Can you work these out from the model? Positions are in its coordinate system, mm. A direction names the side the tool comes from. Coordinates: 2 decimals unless noted, no trailing zeros. Loops run counter-clockwise (first coordinate to the right, second up) from the corner with the lowest first, then second, coordinate; pieces in that order, holes last. Notation, with made-up numbers: (49.5, -4) -> (70.5, -4) arc R18 ccw to (70.5, 29) -> close; hole circle Ø5 at (30.5, 79.25). An arc over 180 degrees is marked (long way). Use one line per item in the form item = value. Start each with the question number.
(1) I'm going to push flat-ended pins straight in: pin 1 (1.2 mm diameter, centred on y = 7, z = 9, fed in from -X); pin 2 (3 mm diameter, centred on x = 7.5, y = 7, fed in from -Z); pin 3 (6.5 mm diameter, centred on x = 0.5, z = -4.5, fed in from +Y) (3 decimals). Where does each tip first touch, or does it pass through?
(2) Imagine slicing it at B-B (x = -6.5). List the corners of the cut face in (y, z) for me (3 decimals).
(3) Imagine slicing it at A-A (y = 2.5). List the corners of the cut face in (x, z) for me, plus the area to 3 significant figures.
(4) On a 3-axis mill with a long thin cutter (end or side, diameter ignored), from which of +Z, -Z, +X, -X, +Y, -Y can I reach the whole of each face in a straight line? I mean faces 1 (the flat face through (8, 7, -4)), 2 (the flat face through (-4, 7, 8)), 3 (the flat face through (-5, 4.825, -3)). Say none if no direction works.
(5) Imagine slicing it at D-D (y = 7.5). List the corners of the cut face in (x, z) for me, plus the area to 3 significant figures.
(6) Imagine slicing it at C-C (z = -7.5). List the corners of the cut face in (x, y) for me (3 decimals).
(7) I need wall thicknesses on line 1 (Z direction, x = -1.75, y = 4.5); line 2 (X direction, y = 3.25, z = -1.25); line 3 (Y direction, x = 6.5, z = 10) (3 decimals). Which ranges of each line are inside material? Lowest first, please. Write a range as [from, to].
(8) Thinking about a two-plate mould opening in X: for faces 4 (the flat face through (-11, 2, 4)), 5 (the flat face through (4, 2, -11)), 6 (the cylindrical face through (-1.2, 2.4, -9.1)), which applies, released by +X, released by -X, zero draft, split by the parting line, or undercut?
```python
from build123d import *

# Parameters (mm, degrees)
SKETCH1_R           = 4
SKETCH1_R_2         = 2
BOSS_EXTRUDE1_DEPTH = 4.825
BOSS_EXTRUDE2_DEPTH = 4


with BuildPart() as part:
    # Sketch1 → Boss-Extrude1 (new body)
    with BuildSketch(Plane(origin=(0, 0, 0), x_dir=(1, 0, 0), z_dir=(0, 1, 0))):
        with BuildLine():
            Line((-11, 0), (-11, -8))
            ThreePointArc((-11, -8), (-10.121320344, -10.121320344), (-8, -11))
            Line((-8, -11), (6, -11))
            ThreePointArc((6, -11), (9.535533906, -9.535533906), (11, -6))
            Line((11, -6), (11, 8))
            ThreePointArc((11, 8), (10.121320344, 10.121320344), (8, 11))
            Line((8, 11), (0, 11))
            ThreePointArc((0, 11), (-7.778174593, 7.778174593), (-11, 0))
        make_face()
        with Locations(Location((0, 0, 0), (0, 0, 270))):  # turned: the seam where the file's is
            Circle(SKETCH1_R, mode=Mode.SUBTRACT)
        with Locations(Location((-7.5, 0, 0), (0, 0, 270))):  # turned: the seam where the file's is
            Circle(SKETCH1_R_2, mode=Mode.SUBTRACT)
        with Locations(Location((0, 7.5, 0), (0, 0, 270))):  # turned: the seam where the file's is
            Circle(SKETCH1_R_2, mode=Mode.SUBTRACT)
    extrude(amount=BOSS_EXTRUDE1_DEPTH)

    # Sketch2 → Boss-Extrude2 (add)
    with BuildSketch(Plane(origin=(0, 4.825, 0), x_dir=(1, 0, 0), z_dir=(0, 1, 0))):
        with BuildLine():
            Line((4, -11), (4, -4))
            Line((4, -4), (11, -4))
            Line((11, -4), (11, 4))
            Line((11, 4), (5.656854249, 4))
            ThreePointArc((5.656854249, 4), (4.023861088, 3.154700538), (3.771236166, 1.333333333))
            ThreePointArc((3.771236166, 1.333333333), (2.828427125, -2.828427125), (-1.333333333, -3.771236166))
            ThreePointArc((-1.333333333, -3.771236166), (-3.154700538, -4.023861088), (-4, -5.656854249))
            Line((-4, -5.656854249), (-4, -11))
            Line((-4, -11), (4, -11))
        make_face()
    extrude(amount=BOSS_EXTRUDE2_DEPTH)


solid = part.part
```
Worked out:
q1.pin_1 = -4
q1.pin_2 = -4
q1.pin_3 = 4.825
q2.outline = (0, -8.874) -> (4.825, -8.874) -> (4.825, -1.732) -> (0, -1.732) -> close; (0, 1.732) -> (4.825, 1.732) -> (4.825, 11) -> (0, 11) -> close
q3.outline = (-11, 0) arc R11 ccw to (0, -11) -> (8, -11) arc R3 ccw to (11, -8) -> (11, 6) arc R5 ccw to (6, 11) -> (-8, 11) arc R3 ccw to (-11, 8) -> close; hole circle Ø4 at (-7.5, 0); hole circle Ø8 at (0, 0); hole circle Ø4 at (0, -7.5)
q3.area = 373 mm2
q4.face_1 = -Z, +X, -X, +Y
q4.face_2 = +Z, -Z, -X, +Y
q4.face_3 = -Z, -X, +Y
q5.outline = (-4, 5.66) arc R2 ccw to (-1.33, 3.77) arc R4 cw to (3.77, -1.33) arc R2 ccw to (5.66, -4) -> (11, -4) -> (11, 4) -> (4, 4) -> (4, 11) -> (-4, 11) -> close
q5.area = 116 mm2
q6.outline = (-8.047, 0) -> (-2, 0) -> (-2, 4.825) -> (-8.047, 4.825) -> close; (2, 0) -> (11, 0) -> (11, 4.825) -> (2, 4.825) -> close
q7.line_1 = [-10.86, -8.47], [-6.53, -3.6], [3.6, 11]
q7.line_2 = [-10.93, -9.06], [-5.94, -3.8], [3.8, 11]
q7.line_3 = [0, 4.825]
q8.face_4 = released by -X
q8.face_5 = zero draft
q8.face_6 = undercut
